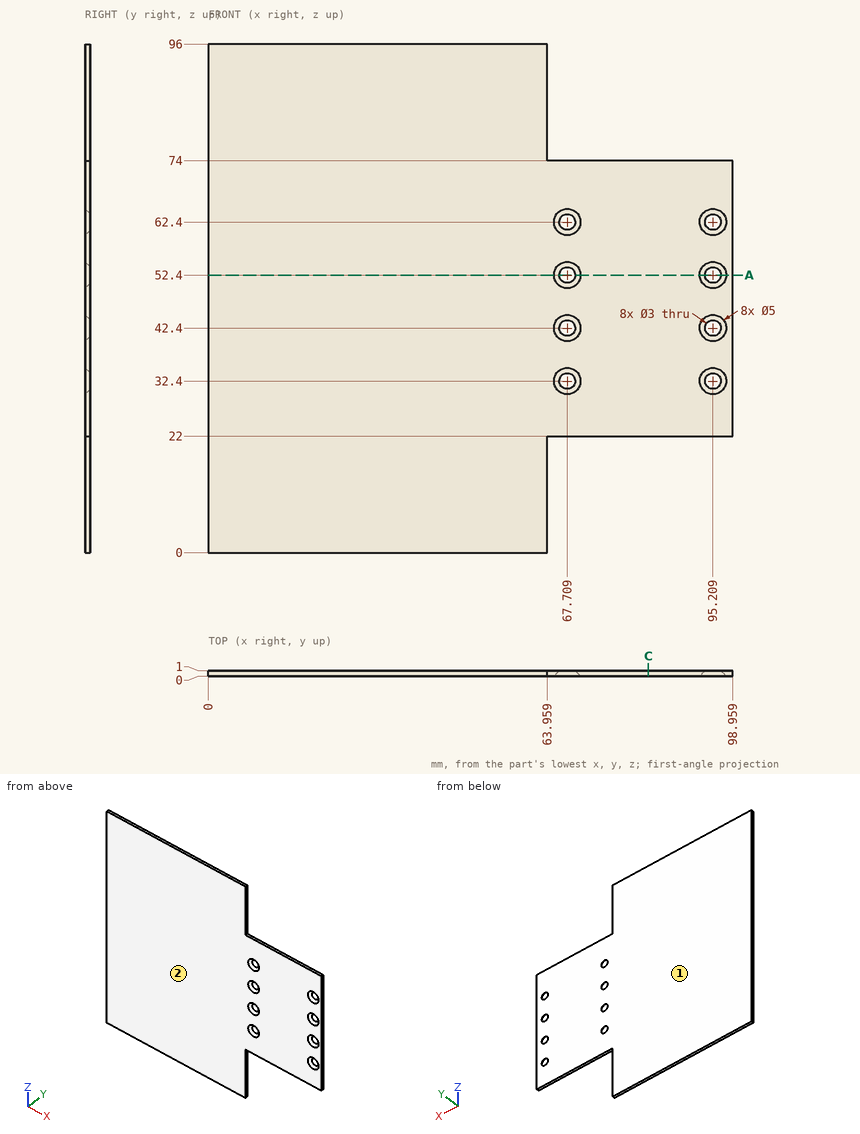
Source: three-view drawing plus pictorial views. Frame: mm from the lowest corner of the part. Give positions to 0.01 mm unless a question says otherwise; leave off trailing zeros. Loops run counter-clockwise (first coordinate to the right, second up) from the corner with the lowest first, then second, coordinate; pieces in that order, holes last.
1) Section query A-A on z = 52.4. Count the separate pieces of the cut face and the enclosed holes in it.
A:
separate pieces: 3
enclosed holes: 0
2) Mould query, pull axis Y, two halves, no side actions, for the marked faces 1 and 2. Classes: released by +Y, released by -Y, zero draft, split by the parting line, or undercut.
A:
face 1: released by +Y
face 2: released by -Y
3) Contact query for flat-ended pins moving along their axis: pin 1 (4 mm diameter, centred on x = 95.21, z = 42.4, fed in from -Y); pin 2 (3.5 mm diameter, centred on x = 95.21, z = 52.4, fed in from -Y). Output: stop coordinate, or through.
A:
pin 1: stops at y = 0.5
pin 2: stops at y = 0.75
4) Section query C-C on x = 83. Return the cut outline in (y, z).
A:
outline: (0, 22) - (1, 22) - (1, 74) - (0, 74) - close
5) Line query: L1, parallel to X at y = 0.45, z = 86.5; L2, parallel to X at y = 0.5, z = 51; L3, parallel to Z at x = 91.5, y = 0.85. Output: solid intervals per line, ascending.
A:
L1: x = 0 to 63.96
L2: x = 0 to 66.28, 69.14 to 93.78, 96.64 to 98.96
L3: z = 22 to 74
